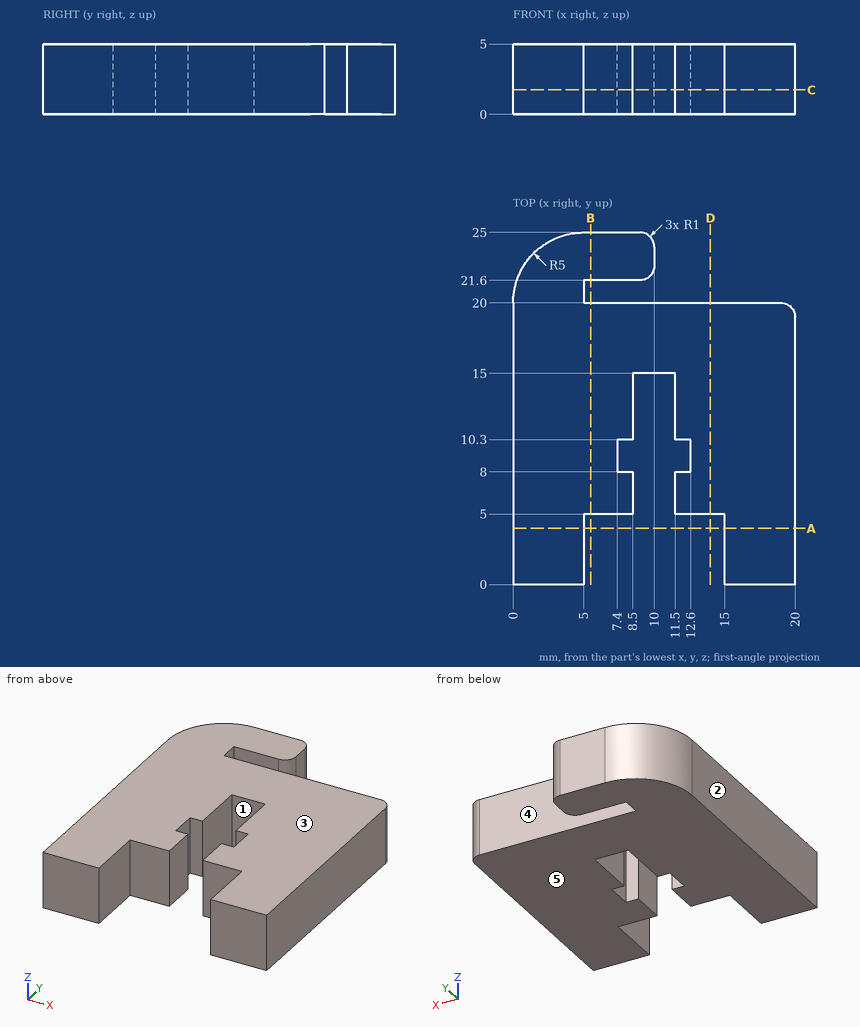
Design review of the part shown in the three views and the two pictorial views. Dimensions are in mm from the part's minimum x, y and z. A direction names the side the tool comes from. Round coordinates to 2 decimals unless told otherwise and drop trailing zeros. Loops run counter-clockwise (first coordinate to the right, second up) from the corner with the lowest first, then second, coordinate; pieces in that order, holes last. Notation, with made-up numbers: (67.25, 74) -> (119.25, 74) arc R17 ccw to (119.25, 101) -> close; hole circle Ø3 at (27, -20.75). An arc over 180 degrees is marked (long way). Answer as a JSON object with one key per item and string values. Group by question number.
1) For line 1 (Y direction, x = 8, z = 4.4); line 2 (X direction, y = 11.5, z = 4.4); line 3 (Y direction, x = 5.75, z = 3), list the stretches that pass through material, from the lowest coordinate up. Write a range as [from, to].
2) We need section A-A on y = 4. Write out the cut boundary in (x, z), then the cut area to 3 significant figures.
3) We need section B-B on x = 5.5. Write out the cut boundary in (y, z).
4) For pin 1 Ø2 at (x, z) = (7, 1.5) entering from -Y; pin 2 Ø0.9 at (x, z) = (10, 2.5) entering from -Y; pin 3 Ø1 at (x, z) = (16, 2.5) entering from +Y; pin 4 Ø1.5 at (x, y) = (5, 6.5) entering from -Z, all flat-tipped, find the tip position at first contact; note any pin that passes through.
5) We need section C-C on z = 1.75. Write out the cut boundary in (x, y), then the cut area to 3 significant figures.
6) Mouldability with a two-part tool opening along Z and no side actions: class the marked faces 3, 4 and 5 as released by +Z, released by -Z, zero draft, split by the parting line, or undercut.
7) For the marked faces 1 and 2, list the 3-axis set-ups (+Z, -Z, +X, -X, +Y, -Y) from which the entire face can be reached by the end or side of a thin tool; tool diameter is ignored.
8) We need section D-D on x = 14. Write out the cut boundary in (y, z).
Result set:
{
 "1": {"line 1": "[5, 8], [10.3, 20], [21.6, 25]", "line 2": "[0, 8.5], [11.5, 20]", "line 3": "[5, 20], [21.6, 25]"},
 "2": {"outline": "(0, 0) -> (5, 0) -> (5, 5) -> (0, 5) -> close; (15, 0) -> (20, 0) -> (20, 5) -> (15, 5) -> close", "area": "50.0 mm²"},
 "3": {"outline": "(5, 0) -> (20, 0) -> (20, 5) -> (5, 5) -> close; (21.6, 0) -> (25, 0) -> (25, 5) -> (21.6, 5) -> close"},
 "4": {"pin 1": "y = 5", "pin 2": "y = 15", "pin 3": "y = 20", "pin 4": "z = 0"},
 "5": {"outline": "(0, 0) -> (5, 0) -> (5, 5) -> (8.5, 5) -> (8.5, 8) -> (7.4, 8) -> (7.4, 10.3) -> (8.5, 10.3) -> (8.5, 15) -> (11.5, 15) -> (11.5, 10.3) -> (12.6, 10.3) -> (12.6, 8) -> (11.5, 8) -> (11.5, 5) -> (15, 5) -> (15, 0) -> (20, 0) -> (20, 19) arc R1 ccw to (19, 20) -> (5, 20) -> (5, 21.6) -> (9, 21.6) arc R1 ccw to (10, 22.6) -> (10, 24) arc R1 ccw to (9, 25) -> (5, 25) arc R5 ccw to (0, 20) -> close", "area": "351 mm²"},
 "6": {"face 3": "released by +Z", "face 4": "zero draft", "face 5": "released by -Z"},
 "7": {"face 1": "+Z, -Z, -Y", "face 2": "+Z, -Z, -X, +Y, -Y"},
 "8": {"outline": "(5, 0) -> (20, 0) -> (20, 5) -> (5, 5) -> close"}
}
